For this review, take the finished solid that the model builds, in its own axes (mm). Coordinates: 2 decimals unless noted, no trailing zeros. Loops run counter-clockwise (first coordinate to the right, second up) from the corner with the lowest first, then second, coordinate; pieces in that order, holes last. Notation, with made-up numbers: (85, 61.5) - (91, 61.5) arc R18 ccw to (91, 89.5) - close; hole circle Ø11 at (48.25, 76). An arc over 180 degrees is marked (long way). One line per item, written item: value. Start each with the question number.
1. Take a section at B-B, the plane x = 20. State the section outline as (y, z) points.
2. To check wall thickness, follow line 1 (X direction, y = 0.2, z = 1); line 2 (Z direction, x = 20, y = 1); line 3 (X direction, y = 0.65, z = -10.5). State the ranges of each line that lie inside material, in increasing order. Write a range as from..to.
3. The part is to be moulded in two halves that separate along Z. For faces 1 (the face through (-18.683, 1.479, 10.942)), 2 (the face through (-18.82, 1.48, -1.08)), 3 (the face through (0, 1, -21.651)), say which applies: released by +Z, released by -Z, zero draft, split by the parting line, or undercut.
4. Take a section at C-C, the plane y = 2.45. State the section outline as (x, z) points.
5. Take a section at A-A, the plane z = 0. State the section outline as (x, y) points, and give its area (3 significant figures).
6. Take a section at D-D, the plane x = -15. State the section outline as (y, z) points.
Autodesk Inventor part; units mm, degrees
ref_plane "YZ Plane" through (0, 0, 0) normal (1, 0, 0) x (0, 1, 0)
ref_plane "XZ Plane" through (0, 0, 0) normal (0, 1, 0) x (-1, 0, 0)
ref_plane "XY Plane" through (0, 0, 0) normal (0, 0, 1) x (1, 0, 0)
sketch "Sketch1" plane through (0, 0, 0) normal (0, 1, 0) x (-1, 0, 0)
  line L0 (23.5566, -2.5) -> (13.9434, -19.1506)
  line L1 (9.6132, -21.6506) -> (-9.6132, -21.6506)
  line L2 (-13.9434, -19.1506) -> (-23.5566, -2.5)
  line L3 (-23.5566, 2.5) -> (-13.9434, 19.1506)
  line L4 (-9.6132, 21.6506) -> (9.6132, 21.6506)
  line L5 (13.9434, 19.1506) -> (23.5566, 2.5)
  line L6 (0, 0) -> (20, 0)
  line L7 (0, 0) -> (-20, 0)
  circle A0 centre (20, 0) radius 1.6
  circle A1 centre (-20, 0) radius 1.6
  arc A2 (13.9434, 19.1506) -> (9.6132, 21.6506) centre (9.6132, 16.6506) ccw
  arc A3 (23.5566, -2.5) -> (23.5566, 2.5) centre (19.2265, 0) ccw
  arc A4 (9.6132, -21.6506) -> (13.9434, -19.1506) centre (9.6132, -16.6506) ccw
  arc A5 (-13.9434, -19.1506) -> (-9.6132, -21.6506) centre (-9.6132, -16.6506) ccw
  arc A6 (-23.5566, 2.5) -> (-23.5566, -2.5) centre (-19.2265, 0) ccw
  arc A7 (-9.6132, 21.6506) -> (-13.9434, 19.1506) centre (-9.6132, 16.6506) ccw
  point P0 (25, 0)
  point P1 (12.5, -21.6506)
  point P2 (-12.5, -21.6506)
  point P3 (-25, 0)
  point P4 (-12.5, 21.6506)
  point P5 (12.5, 21.6506)
  dimension "d0" = 50
  dimension "d1" = 20
  dimension "d2" = 20
  dimension "d3" = 3.2
  dimension "d4" = 3.2
  dimension "d5" = 5
extrude "Extrusion1" add sketch "Sketch1" along normal blind 3
properties part number "Battery cover hex"
Solutions:
1. outline: (0, -8.66) - (3, -8.66) - (3, -1.6) - (0, -1.6) - close; (0, 1.6) - (3, 1.6) - (3, 8.66) - (0, 8.66) - close
2. line 1: -24.13..-21.25, -18.75..18.75, 21.25..24.13
2. line 2: -8.66..-1.6, 1.6..8.66
2. line 3: -18.94..18.94
3. face 1: released by +Z
3. face 2: undercut
3. face 3: released by -Z
4. outline: (-23.56, -2.5) - (-13.94, -19.15) arc R5 ccw to (-9.61, -21.65) - (9.61, -21.65) arc R5 ccw to (13.94, -19.15) - (23.56, -2.5) arc R5 ccw to (23.56, 2.5) - (13.94, 19.15) arc R5 ccw to (9.61, 21.65) - (-9.61, 21.65) arc R5 ccw to (-13.94, 19.15) - (-23.56, 2.5) arc R5 ccw to start; hole circle Ø3.2 at (-20, 0); hole circle Ø3.2 at (20, 0)
5. outline: (-24.23, 0) - (-21.6, 0) - (-21.6, 3) - (-24.23, 3) - close; (-18.4, 0) - (18.4, 0) - (18.4, 3) - (-18.4, 3) - close; (21.6, 0) - (24.23, 0) - (24.23, 3) - (21.6, 3) - close
5. area: 126 mm2
6. outline: (0, -17.32) - (3, -17.32) - (3, 17.32) - (0, 17.32) - close
